Geometry check sheet. Reference: drawing and pictorial views, mm from the part's lowest x, y, z. A direction names the side the tool comes from. Coordinates: 2 decimals unless noted, no trailing zeros. Loops run counter-clockwise (first coordinate to the right, second up) from the corner with the lowest first, then second, coordinate; pieces in that order, holes last. Notation, with made-up numbers: (-16.5, 11) - (-10.5, 11) arc R21 ccw to (-10.5, 22) - close; hole circle Ø9 at (42, -39.5). An arc over 180 degrees is marked (long way). Use a Markdown table: item, result. Add a question column.
1) Sectioned sample at B-B, the plane x = 119. Enter the section's corners in (y, z) (1 decimal).
2) Draft check along X on the marked faces 3, 4, 5 and 6. Enter one of: pulls with the +X half, pulls with the -X half, needs draft (parallel to the pull), parting line crosses it, or undercut.
3) Sectioned sample at D-D, the plane z = 90. Enter the section's corners in (x, y) (1 decimal).
4) Thickness scan on line 1 (X direction, y = 7.25, z = 88.9); line 2 (Z direction, x = 106.5, y = 28) (1 decimal). Record the ranges inside material, lowest first.
5) Go/stop test with flat-tipped pins: P1, Ø22, axis at x = 88.9, z = 20.64, coming from the +Y side (1 decimal); P2, Ø8, axis at y = 25, z = 103.5, coming from the -X side (1 decimal); P3, Ø12.5, axis at y = 36, z = 106, coming from the +X side (1 decimal). Record where each tip stops, or that it passes through.
6) Sectioned sample at C-C, the plane y = 43. Enter the section's corners in (x, z) (1 decimal), then the cut area to 3 significant figures.
7) Tool access check on the marked faces 1 and 2. Record the directions out of +Z, -Z, +X, -X, +Y, -Y that give a thin tool (end or side, any length) a straight path to the whole face; none if there is none.
8) Sectioned sample at A-A, the plane z = 70. Enter the section's corners in (x, y) (1 decimal), then the cut area to 3 significant figures.
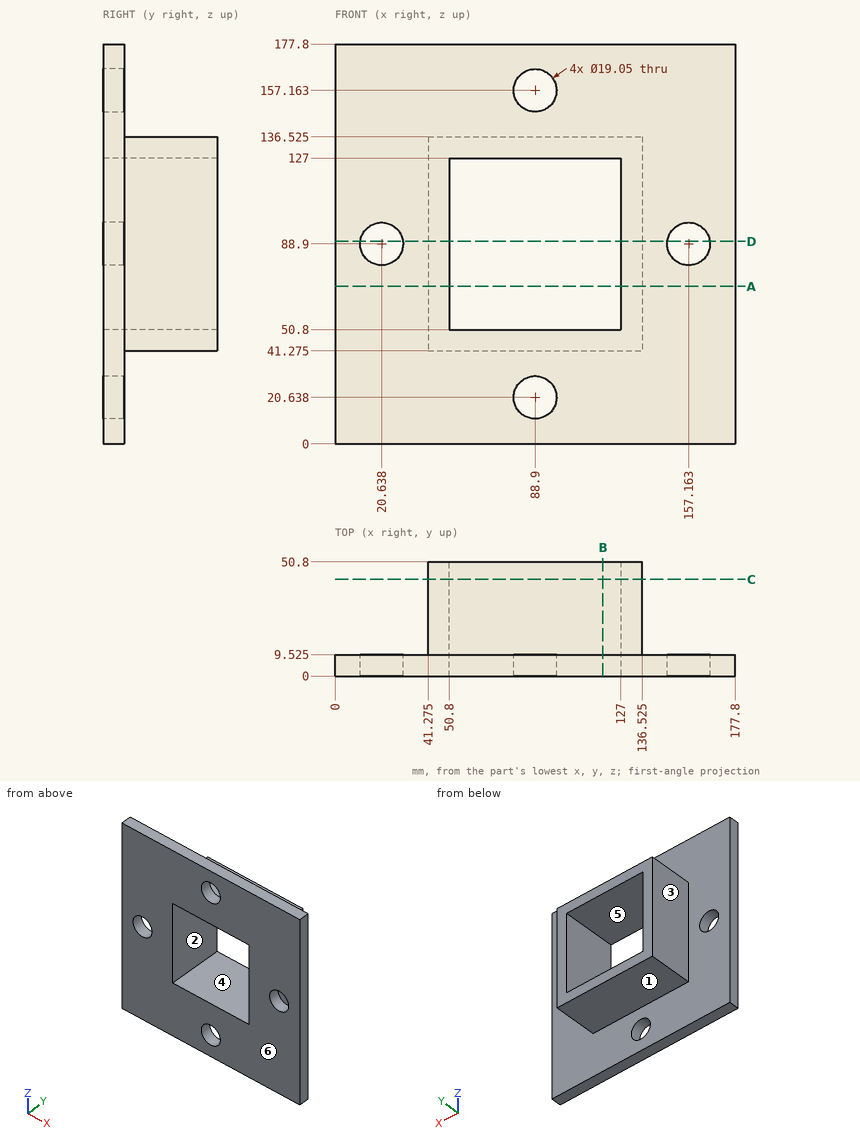
Solved:
| question | item | result |
|---|---|---|
| 1 | outline | (0, 0) - (9.5, 0) - (9.5, 41.3) - (50.8, 41.3) - (50.8, 50.8) - (0, 50.8) - close; (0, 127) - (50.8, 127) - (50.8, 136.5) - (9.5, 136.5) - (9.5, 177.8) - (0, 177.8) - close |
| 2 | face 3 | pulls with the -X half |
| 2 | face 4 | undercut |
| 2 | face 5 | undercut |
| 2 | face 6 | needs draft |
| 3 | outline | (0, 0) - (11.2, 0) - (11.2, 9.5) - (0, 9.5) - close; (30.1, 0) - (50.8, 0) - (50.8, 50.8) - (41.3, 50.8) - (41.3, 9.5) - (30.1, 9.5) - close; (127, 0) - (147.7, 0) - (147.7, 9.5) - (136.5, 9.5) - (136.5, 50.8) - (127, 50.8) - close; (166.6, 0) - (177.8, 0) - (177.8, 9.5) - (166.6, 9.5) - close |
| 4 | line 1 | x = 0 to 11.11, 30.16 to 50.8, 127 to 147.64, 166.69 to 177.8 |
| 4 | line 2 | z = 41.3 to 50.8, 127 to 136.5 |
| 5 | P1 | stops at y = 9.5 |
| 5 | P2 | stops at x = 41.3 |
| 5 | P3 | stops at x = 136.5 |
| 6 | outline | (41.3, 41.3) - (136.5, 41.3) - (136.5, 136.5) - (41.3, 136.5) - close; hole (50.8, 50.8) - (127, 50.8) - (127, 127) - (50.8, 127) - close |
| 6 | area | 3,270 mm2 |
| 7 | face 1 | -Z, +X, -X, +Y |
| 7 | face 2 | +Y, -Y |
| 8 | outline | (0, 0) - (50.8, 0) - (50.8, 50.8) - (41.3, 50.8) - (41.3, 9.5) - (0, 9.5) - close; (127, 0) - (177.8, 0) - (177.8, 9.5) - (136.5, 9.5) - (136.5, 50.8) - (127, 50.8) - close |
| 8 | area | 1,750 mm2 |
